from build123d import *

# Parameters (mm, degrees)
F0_R     = 1
F1_DEPTH = 1.25


with BuildPart() as f1:
    # F0 (on Top) → F1 (new body)
    with BuildSketch(Plane.XY):
        with BuildLine():
            Line((5.178727, -3.631317), (1.810287, 2.39225))
            ThreePointArc((1.810287, 2.39225), (0.95479, 2.844007), (0, 3))
            Line((0, 3), (-30, 3))
            Line((-30, 3), (-30, -1.74156))
            Line((-30, -1.74156), (-3.909058, -1.74156))
            ThreePointArc((-3.909058, -1.74156), (-2.644244, -2.085117), (-1.727059, -3.021363))
            Line((-1.727059, -3.021363), (-0.093587, -5.942397))
            Line((-0.093587, -5.942397), (3.094821, -5.942397))
            Line((3.094821, -5.942397), (4.794006, -4.992196))
            ThreePointArc((4.794006, -4.992196), (5.268214, -4.391435), (5.178727, -3.631317))
        make_face()
        Circle(F0_R, mode=Mode.SUBTRACT)
    extrude(amount=F1_DEPTH)


solid = f1.part
For this review, take the finished solid that the model builds, in its own axes (mm). A direction names the side the tool comes from. Coordinates: 2 decimals unless noted, no trailing zeros. Order: outer loops, then holes, each group sorted by start corner. A loop starts at its lowest first (then second) coordinate and runs counter-clockwise, first axis right, second up. Notation, with made-up numbers: (39, -7) - (98, -7) arc R24 cw to (98, 29) - close; hole circle Ø6 at (60.5, -3.75). An arc over 180 degrees is marked (long way). Answer as CSV lines item,"result". Start each with the question number.
1) Add section A-A (z = 0.2). State the section outline as (x, y) points, then the cut area to 3 significant figures.
2) Insertion check: P1, Ø4, axis at x = -13.5, y = -2.5, coming from the -Z side; P2, Ø1.6, axis at x = 0, y = 0, coming from the -Z side. Each pin has a flat end and moves straight along its axis. Give the tip position at first contact, or say it passes through.
3) Add section B-B (y = 0). State the section outline as (x, z) points.
4) Add section D-D (y = -5.5). State the section outline as (x, z) points.
5) Machinability: for faces 4 (the flat face through (-17, -1.742, 1)), 5 (the cylindrical face through (5.265, -4.402, 0.616)), which of the approach directions +Z, -Z, +X, -X, +Y, -Y give a long, thin tool a straight path to every point of the face, cutting with its end or side? Answer none if there is none.
6) Add section C-C (x = -5.5). State the section outline as (y, z) points.
7) To check wall thickness, follow line 1 along Y through (x, z) = (-17.5, 0.9); line 2 along X through (y, z) = (-3.75, 0.25); line 3 along X through (y, z) = (-2.75, 0.1). State the ranges of each line that lie inside material, in increasing order. Write a range as [from, to].
8) Draft analysis for pull direction X (two halves, no side actions). For faces 1 (the flat face through (3.518, -0.662, 0.616)), 2 (the flat face through (-0.9, -4.5, 0.6)), 3 (the cylindrical face through (0, -1, 1)), state which applies: +X half, -X half, draft (parallel to the pull), parting line (faces both ways), or undercut.
Result:
1,outline,"(-30, -1.74) - (-3.91, -1.74) arc R2.5 cw to (-1.73, -3.02) - (-0.09, -5.94) - (3.09, -5.94) - (4.79, -4.99) arc R1 ccw to (5.18, -3.63) - (1.81, 2.39) arc R3 ccw to (0, 3) - (-30, 3) - close; hole circle Ø2 at (0, 0)"
1,area,"177 mm^2"
2,P1,"z = 0"
2,P2,"through"
3,outline,"(-30, 0) - (-1, 0) - (-1, 1.25) - (-30, 1.25) - close; (1, 0) - (3.15, 0) - (3.15, 1.25) - (1, 1.25) - close"
4,outline,"(-0.34, 0) - (3.89, 0) - (3.89, 1.25) - (-0.34, 1.25) - close"
5,face 4,"+Z, -Z, -X, -Y"
5,face 5,"+Z, -Z, +X"
6,outline,"(-1.74, 0) - (3, 0) - (3, 1.25) - (-1.74, 1.25) - close"
7,line 1,"[-1.74, 3]"
7,line 2,"[-1.32, 5.24]"
7,line 3,"[-1.9, 4.69]"
8,face 1,"+X half"
8,face 2,"-X half"
8,face 3,"undercut"
